Source: CAD feature listing. Evaluate the final solid. Frame: model axes, mm. Face numbers are marked on the shaded views. A direction names the side the tool comes from. Give positions to 0.01 mm unless a question says otherwise; leave off trailing zeros. Loops run counter-clockwise (first coordinate to the right, second up) from the corner with the lowest first, then second, coordinate; pieces in that order, holes last. Notation, with made-up numbers: M 67.25,-37 L 119.25,-37 A25 ccw 119.25,2 Z; hole C 77,-9.75 d6. An arc over 180 degrees is marked long. Answer in a Markdown table with one row per item.
```python
from build123d import *

# Parameters (mm, degrees)
SKETCH_1_W      = 100
SKETCH_1_H      = 35
EXTRUDE_1_DEPTH = 5
SKETCH_3_W      = 50
SKETCH_3_H      = 11
EXTRUDE_2_DEPTH = 5


with BuildPart() as part:
    # 草图1 → 凸台-拉伸1 (new body)
    with BuildSketch(Plane(origin=(0, 0, 0), x_dir=(1, 0, 0), z_dir=(0, 1, 0))):
        Rectangle(SKETCH_1_W, SKETCH_1_H)
    extrude(amount=EXTRUDE_1_DEPTH)

    # 草图3 → 凸台-拉伸2 (add, symmetric)
    with BuildSketch(Plane(origin=(0, 0, 0), x_dir=(0, 0, -1), z_dir=(1, 0, 0))):
        with Locations((0, 2.5)):
            Rectangle(SKETCH_3_W, SKETCH_3_H)
    extrude(amount=EXTRUDE_2_DEPTH, both=True)


solid = part.part
```
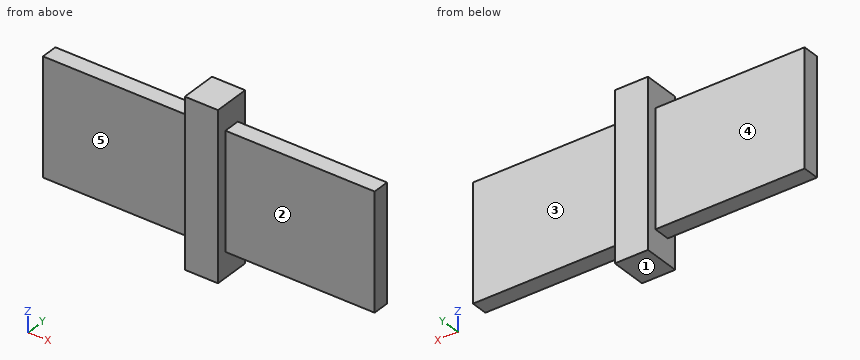
1) Section D-D, the plane z = 19.5. Return loops of the section in (x, y), then the cut area to 3 significant figures.
Reply:
| item | result |
|---|---|
| outline | M -5,-3 L 5,-3 L 5,8 L -5,8 Z |
| area | 110 mm² |
2) Pin query (flat end, axial travel): pin 1 Ø10.5 at (x, z) = (28.5, 6) entering from +Y; pin 2 Ø4 at (x, y) = (-28.5, 3) entering from +Z; pin 3 Ø1 at (y, z) = (6.5, -13) entering from -X. Return the tip coordinate at first contact, or that it passes through.
Reply:
| item | result |
|---|---|
| pin 1 | stops at y = 5 |
| pin 2 | stops at z = 17.5 |
| pin 3 | stops at x = -5 |
3) Set-up query: the marked faces 1, 2, 3, 4 and 5. Return all of +Z, -Z, +X, -X, +Y, -Y with unobstructed straight access to the full face (end or side cutting, diameter ignored); none if empty.
Reply:
| item | result |
|---|---|
| face 1 | -Z, +X, -X, +Y, -Y |
| face 2 | +Z, -Z, +X, -Y |
| face 3 | +Z, -Z, +X, +Y |
| face 4 | +Z, -Z, -X, +Y |
| face 5 | +Z, -Z, -X, -Y |
4) Material intervals for L1, parallel to Y at x = 35, z = -14.5; L2, parallel to X at y = 5.5, z = -5; L3, parallel to Z at x = -25.5, y = 3.5, sorted ascending.
Reply:
| item | result |
|---|---|
| L1 | y = 0 to 5 |
| L2 | x = -5 to 5 |
| L3 | z = -17.5 to 17.5 |
5) Section A-A, the plane z = -1. Return loops of the section in (x, y).
Reply:
| item | result |
|---|---|
| outline | M -50,0 L -5,0 L -5,-3 L 5,-3 L 5,0 L 50,0 L 50,5 L 5,5 L 5,8 L -5,8 L -5,5 L -50,5 Z |
6) Section B-B, the plane y = 1.25. Return loops of the section in (x, z), then the cut area to 3 significant figures.
Reply:
| item | result |
|---|---|
| outline | M -50,-17.5 L -5,-17.5 L -5,-25 L 5,-25 L 5,-17.5 L 50,-17.5 L 50,17.5 L 5,17.5 L 5,25 L -5,25 L -5,17.5 L -50,17.5 Z |
| area | 3,650 mm² |
7) Section C-C, the plane x = 30. Return loops of the section in (y, z).
Reply:
| item | result |
|---|---|
| outline | M 0,-17.5 L 5,-17.5 L 5,17.5 L 0,17.5 Z |
